Can you work these out from the model? Positions are in its coordinate system, mm. A direction names the side the tool comes from. Round coordinates to 2 decimals unless told otherwise and drop trailing zeros. Write each loop counter-clockwise with the first axis right and the second up, starting at its lowest first coordinate (ties: lowest second). Pieces come first, ordered by that corner, then holes. Notation, with made-up numbers: (37, 84) - (61, 84) arc R30 cw to (61, 113) - close; hole circle Ø5 at (28.25, 77). An arc over 180 degrees is marked (long way). One line per item, written item: value. Start each with the question number.
(1) I want a section at C-C on z = -3. List the corners of the cut face in (x, y) for me.
(2) Thinking about a two-plate mould opening in Z: for faces 1 (the face through (0, 22.3, -12)), 2 (the face through (0, 44.5, -6)), which applies, +Z half, -Z half, draft (parallel to the pull), parting line (faces both ways), or undercut?
(3) I want a section at D-D on x = -15. List the corners of the cut face in (y, z) for me.
(4) If I drill on L1, parallel to Z at x = 24.75, y = -18.1; L2, parallel to Y at x = -15, z = -11.5; L3, parallel to Z at x = -14, y = 10, over which ranges is the centre line in solid material (lowest first)? Write a range as from..to.
(5) I want a section at B-B on x = -24.75. List the corners of the cut face in (y, z) for me, plus the area to 3 significant figures.
(6) I'm going to push flat-ended pins straight in: pin 1 Ø1.6 at (x, z) = (26.5, -24) entering from +Y; pin 2 Ø5 at (x, z) = (1.5, -12.5) entering from +Y; pin 3 Ø8 at (x, z) = (-24.5, -11.5) entering from +Y. Where does each tip first touch, or does it pass through?
(7) On a 3-axis mill with a long thin cutter (end or side, diameter ignored), from which of +Z, -Z, +X, -X, +Y, -Y can I reach the whole of each face in a straight line? I mean faces 3 (the face through (-25, 2.5, 1)), 4 (the face through (0, 17.5, -12)), 5 (the face through (20, 28, -11)). Say none if no direction works.
(8) I want a section at A-A on y = 7. List the corners of the cut face in (x, z) for me, plus the area to 3 significant figures.
from build123d import *

# Parameters (mm, degrees)
SKETCH_1_W          = 10
SKETCH_1_H          = 20
SKETCH_1_W_2        = 40
SKETCH_1_H_2        = 35
EXTRUDE_1_DEPTH     = 2
SKETCH_3_W          = 10
SKETCH_3_H          = 25
EXTRUDE_2_DEPTH     = 2
EXTRUDE_3_DEPTH     = 2
CUT_EXTRUDE_1_REACH = 54.44
SKETCH_5_R          = 2.1
EXTRUDE_5_DEPTH     = 2
SKETCH_7_W          = 40
SKETCH_7_H          = 27
EXTRUDE_6_DEPTH     = 25
CUT_EXTRUDE_2_REACH = 73.451
SKETCH_8_R          = 2.6
SKETCH_9_W          = 15
SKETCH_9_H          = 10.5
CUT_EXTRUDE_3_DEPTH = 22.2


with BuildPart() as part:
    # 草图1 → 凸台-拉伸1 (new body)
    with BuildSketch(Plane.XY):
        with Locations((-25, -7.5)):
            Rectangle(SKETCH_1_W, SKETCH_1_H)
        Rectangle(SKETCH_1_W_2, SKETCH_1_H_2)
        with Locations((25, -7.5)):
            Rectangle(SKETCH_1_W, SKETCH_1_H)
    extrude(amount=EXTRUDE_1_DEPTH)

    # 草图3 → 凸台-拉伸2 (add)
    with BuildSketch(Plane.XZ.offset(17.5)):
        with Locations((-25, -10.5)):
            Rectangle(SKETCH_3_W, SKETCH_3_H)
        with Locations((25, -10.5)):
            Rectangle(SKETCH_3_W, SKETCH_3_H)
    extrude(amount=EXTRUDE_2_DEPTH)

    # 草图4 → 凸台-拉伸3 (add)
    with BuildSketch(Plane(origin=(0, 0, -23), x_dir=(-1, 0, 0), z_dir=(0, 0, -1))):
        Polygon((30, -19.5), (30, -17.5), (30, 2.5), (20, 2.5), (20, 17.5), (-20, 17.5), (-20, 2.5), (-30, 2.5), (-30, -17.5), (-30, -19.5), align=None)
    extrude(amount=EXTRUDE_3_DEPTH)

    # 草图5 → 切除-拉伸1 (cut, up to next)
    with BuildSketch(Plane(origin=(0, -17.5, 0), x_dir=(1, 0, 0), z_dir=(0, 1, 0)), mode=Mode.PRIVATE) as cut_extrude_1_sk1:
        with Locations(Location((24.75, 16.5, 0), (0, 0, 180))):
            Circle(SKETCH_5_R)
    cut_extrude_1_tool1 = extrude(cut_extrude_1_sk1.sketch, amount=-CUT_EXTRUDE_1_REACH, mode=Mode.PRIVATE) & part.part
    # 草图5 → 切除-拉伸1 (cut, up to next)
    with BuildSketch(Plane(origin=(0, -17.5, 0), x_dir=(1, 0, 0), z_dir=(0, 1, 0)), mode=Mode.PRIVATE) as cut_extrude_1_sk2:
        with Locations(Location((24.75, 6.5, 0), (0, 0, 180))):
            Circle(SKETCH_5_R)
    cut_extrude_1_tool2 = extrude(cut_extrude_1_sk2.sketch, amount=-CUT_EXTRUDE_1_REACH, mode=Mode.PRIVATE) & part.part
    # 草图5 → 切除-拉伸1 (cut, up to next)
    with BuildSketch(Plane(origin=(0, -17.5, 0), x_dir=(1, 0, 0), z_dir=(0, 1, 0)), mode=Mode.PRIVATE) as cut_extrude_1_sk3:
        with Locations(Location((-24.75, 16.5, 0), (0, 0, 180))):
            Circle(SKETCH_5_R)
    cut_extrude_1_tool3 = extrude(cut_extrude_1_sk3.sketch, amount=-CUT_EXTRUDE_1_REACH, mode=Mode.PRIVATE) & part.part
    # 草图5 → 切除-拉伸1 (cut, up to next)
    with BuildSketch(Plane(origin=(0, -17.5, 0), x_dir=(1, 0, 0), z_dir=(0, 1, 0)), mode=Mode.PRIVATE) as cut_extrude_1_sk4:
        with Locations(Location((-24.75, 6.5, 0), (0, 0, 180))):
            Circle(SKETCH_5_R)
    cut_extrude_1_tool4 = extrude(cut_extrude_1_sk4.sketch, amount=-CUT_EXTRUDE_1_REACH, mode=Mode.PRIVATE) & part.part
    add(cut_extrude_1_tool1.solids().sort_by_distance((24.75, -17.5, -16.5))[0], mode=Mode.SUBTRACT)
    add(cut_extrude_1_tool2.solids().sort_by_distance((24.75, -17.5, -6.5))[0], mode=Mode.SUBTRACT)
    add(cut_extrude_1_tool3.solids().sort_by_distance((-24.75, -17.5, -16.5))[0], mode=Mode.SUBTRACT)
    add(cut_extrude_1_tool4.solids().sort_by_distance((-24.75, -17.5, -6.5))[0], mode=Mode.SUBTRACT)

    # 草图6 → 凸台-拉伸5 (add)
    with BuildSketch(Plane(origin=(0, 17.5, 0), x_dir=(1, 0, 0), z_dir=(0, 1, 0))):
        Polygon((-20, 0), (-20, -2), (20, -2), (20, 0), (20, 23), (20, 25), (-20, 25), (-20, 23), align=None)
    extrude(amount=EXTRUDE_5_DEPTH)

    # 草图7 → 凸台-拉伸6 (add)
    with BuildSketch(Plane(origin=(0, 19.5, 0), x_dir=(1, 0, 0), z_dir=(0, 1, 0))):
        with Locations((0, 11.5)):
            Rectangle(SKETCH_7_W, SKETCH_7_H)
    extrude(amount=EXTRUDE_6_DEPTH)

    # 草图8 → 切除-拉伸2 (cut, up to next)
    with BuildSketch(Plane.ZY.offset(20), mode=Mode.PRIVATE) as cut_extrude_2_sk1:
        with Locations((-11.5, 32.5)):
            Circle(SKETCH_8_R)
    cut_extrude_2_tool1 = extrude(cut_extrude_2_sk1.sketch, amount=-CUT_EXTRUDE_2_REACH, mode=Mode.PRIVATE) & part.part
    add(cut_extrude_2_tool1.solids().sort_by_distance((-20, 32.5, -11.5))[0], mode=Mode.SUBTRACT)

    # 草图9 → 切除-拉伸3 (cut)
    with BuildSketch(Plane(origin=(0, 44.5, 0), x_dir=(1, 0, 0), z_dir=(0, 1, 0))):
        with Locations((0, 11.5)):
            Rectangle(SKETCH_9_W, SKETCH_9_H)
    extrude(amount=-CUT_EXTRUDE_3_DEPTH, mode=Mode.SUBTRACT)


solid = part.part
Established:
1. outline: (-30, -19.5) - (-20, -19.5) - (-20, -17.5) - (-30, -17.5) - close; (-20, 17.5) - (20, 17.5) - (20, 44.5) - (-20, 44.5) - close; (20, -19.5) - (30, -19.5) - (30, -17.5) - (20, -17.5) - close
2. face 1: undercut
2. face 2: draft
3. outline: (-19.5, -25) - (44.5, -25) - (44.5, 2) - (-17.5, 2) - (-17.5, 0) - (17.5, 0) - (17.5, -23) - (-19.5, -23) - close; hole circle Ø5.2 at (32.5, -11.5)
4. L1: -25..-18.6, -14.4..-8.6, -4.4..2
4. L2: 17.5..29.9, 35.1..44.5
4. L3: -25..-23, 0..2
5. outline: (-19.5, -25) - (2.5, -25) - (2.5, -23) - (-17.5, -23) - (-17.5, -18.6) - (-19.5, -18.6) - close; (-19.5, -14.4) - (-17.5, -14.4) - (-17.5, -8.6) - (-19.5, -8.6) - close; (-19.5, -4.4) - (-17.5, -4.4) - (-17.5, 0) - (2.5, 0) - (2.5, 2) - (-19.5, 2) - close
5. area: 117 mm2
6. pin 1: y = 2.5
6. pin 2: y = 22.3
6. pin 3: y = -17.5
7. face 3: +Z, -Z, -X, +Y
7. face 4: +X, -X, -Y
7. face 5: +Z, -Z, +X, +Y
8. outline: (-20, -25) - (20, -25) - (20, -23) - (-20, -23) - close; (-20, 0) - (20, 0) - (20, 2) - (-20, 2) - close
8. area: 160 mm2
